```python
from build123d import *

# Parameters (mm, degrees)
SKETCH1_W                            = 26.5
SKETCH1_H                            = 6
BOSS_EXTRUDE1_DEPTH                  = 17
SKETCH2_R                            = 1.5
CUT_EXTRUDE1_DEPTH                   = 1
SKETCH3_R                            = 1.3
CUT_EXTRUDE2_DEPTH                   = 32.878676259
SKETCH4_R                            = 3
CUT_EXTRUDE3_DEPTH                   = 33.050741021
SKETCH5_R                            = 2.5
CUT_EXTRUDE4_DEPTH                   = 1.5
SKETCH6_R                            = 1.5
CUT_EXTRUDE8_DEPTH                   = 1
SKETCH7_R                            = 1.3
CUT_EXTRUDE9_DEPTH                   = 32.678068123
CUT_EXTRUDE10_START                  = -1
SKETCH8_R                            = 2.5
CUT_EXTRUDE10_DEPTH                  = 1
CUT_EXTRUDE11_START                  = -1
SKETCH9_R                            = 1.5
CUT_EXTRUDE11_DEPTH                  = 1
SKETCH10_R                           = 5.5
SKETCH10_R_2                         = 3
BOSS_EXTRUDE2_DEPTH                  = 3.5
SKETCH11_R                           = 3
SKETCH11_R_2                         = 1.3
BOSS_EXTRUDE4_DEPTH                  = 2
CUT_EXTRUDE12_START                  = -1
SKETCH12_R                           = 1.5
CUT_EXTRUDE12_DEPTH                  = 1
SKETCH17_W                           = 2
SKETCH17_H                           = 6
BOSS_EXTRUDE6_DEPTH                  = 1.5
SKETCH18_R                           = 1
CUT_EXTRUDE17_DEPTH                  = 33.050741021
CHAMFER2_SIZE                        = 5
CHAMFER2_SIZE2                       = 3.5
FILLET11_R                           = 3
BOSS_EXTRUDE7_DEPTH                  = 2
CUT_EXTRUDE19_DEPTH                  = 33.050741021
FILLET13_R                           = 5
FILLET14_R                           = 3
FILLET15_R                           = 3
SKIZZE1_R                            = 1
SCHNITT_LINEAR_AUSTRAGEN1_DEPTH      = 33.050741021
SCHNITT_LINEAR_AUSTRAGEN2_DEPTH      = 31.409702399
SCHNITT_LINEAR_AUSTRAGEN2_DEPTH_BACK = 31.409702399
SKIZZE2_W                            = 26.5
SKIZZE2_H                            = 3


with BuildPart() as part:
    # Sketch1 → Boss-Extrude1 (new body)
    with BuildSketch(Plane(origin=(0, 0, 0), x_dir=(1, 0, 0), z_dir=(0, 1, 0))):
        with Locations((13.25, 3)):
            Rectangle(SKETCH1_W, SKETCH1_H)
    extrude(amount=BOSS_EXTRUDE1_DEPTH)

    # Sketch2 → Cut-Extrude1 (cut)
    with BuildSketch(Plane.XY):
        with Locations((12.5, 5.5)):
            Circle(SKETCH2_R)
    extrude(amount=-CUT_EXTRUDE1_DEPTH, mode=Mode.SUBTRACT)

    # Sketch3 → Cut-Extrude2 (cut, through all)
    with BuildSketch(Plane.XY.offset(-1)):
        with Locations((12.5, 5.5)):
            Circle(SKETCH3_R)
    extrude(amount=-CUT_EXTRUDE2_DEPTH, mode=Mode.SUBTRACT)

    # Sketch4 → Cut-Extrude3 (cut, through all)
    with BuildSketch(Plane.XY):
        with Locations((19.208203932, 11.5)):
            Circle(SKETCH4_R)
    extrude(amount=-CUT_EXTRUDE3_DEPTH, mode=Mode.SUBTRACT)

    # Sketch5 → Cut-Extrude4 (cut)
    with BuildSketch(Plane.XY):
        with Locations((3.5, 5.5)):
            Circle(SKETCH5_R)
    extrude(amount=-CUT_EXTRUDE4_DEPTH, mode=Mode.SUBTRACT)

    # Sketch6 → Cut-Extrude8 (cut)
    with BuildSketch(Plane.XY.offset(-1.5)):
        with Locations((3.5, 5.5)):
            Circle(SKETCH6_R)
    extrude(amount=-CUT_EXTRUDE8_DEPTH, mode=Mode.SUBTRACT)

    # Sketch7 → Cut-Extrude9 (cut, through all)
    with BuildSketch(Plane.XY.offset(-2.5)):
        with Locations((3.5, 5.5)):
            Circle(SKETCH7_R)
    extrude(amount=-CUT_EXTRUDE9_DEPTH, mode=Mode.SUBTRACT)

    # Sketch8 → Cut-Extrude10 (cut)
    with BuildSketch(Plane(origin=(0, 0, -6), x_dir=(-1, 0, 0), z_dir=(0, 0, -1)).offset(CUT_EXTRUDE10_START)):
        with Locations(Location((-3.5, 5.5, 0), (0, 0, 180))):
            Circle(SKETCH8_R)
    extrude(amount=CUT_EXTRUDE10_DEPTH, mode=Mode.SUBTRACT)

    # Sketch9 → Cut-Extrude11 (cut)
    with BuildSketch(Plane(origin=(0, 0, -5), x_dir=(-1, 0, 0), z_dir=(0, 0, -1)).offset(CUT_EXTRUDE11_START)):
        with Locations(Location((-3.5, 5.5, 0), (0, 0, 180))):
            Circle(SKETCH9_R)
    extrude(amount=CUT_EXTRUDE11_DEPTH, mode=Mode.SUBTRACT)

    # Sketch10 → Boss-Extrude2 (add)
    with BuildSketch(Plane(origin=(0, 0, -6), x_dir=(-1, 0, 0), z_dir=(0, 0, -1))):
        with Locations(Location((-19.208203932, 11.5, 0), (0, 0, 90))):
            Circle(SKETCH10_R)
        with Locations(Location((-19.208203932, 11.5, 0), (0, 0, 180))):
            Circle(SKETCH10_R_2, mode=Mode.SUBTRACT)
    extrude(amount=BOSS_EXTRUDE2_DEPTH)

    # Sketch11 → Boss-Extrude4 (add)
    with BuildSketch(Plane(origin=(0, 0, -6), x_dir=(-1, 0, 0), z_dir=(0, 0, -1))):
        with Locations(Location((-12.5, 5.5, 0), (0, 0, 180))):
            Circle(SKETCH11_R)
        with Locations(Location((-12.5, 5.5, 0), (0, 0, 180))):
            Circle(SKETCH11_R_2, mode=Mode.SUBTRACT)
    extrude(amount=BOSS_EXTRUDE4_DEPTH)

    # Sketch12 → Cut-Extrude12 (cut)
    with BuildSketch(Plane(origin=(0, 0, -8), x_dir=(-1, 0, 0), z_dir=(0, 0, -1)).offset(CUT_EXTRUDE12_START)):
        with Locations(Location((-12.5, 5.5, 0), (0, 0, 180))):
            Circle(SKETCH12_R)
    extrude(amount=CUT_EXTRUDE12_DEPTH, mode=Mode.SUBTRACT)

    # Sketch17 → Boss-Extrude6 (add)
    with BuildSketch(Plane.XZ):
        with Locations((6, -3)):
            Rectangle(SKETCH17_W, SKETCH17_H)
        with Locations((20.5, -3)):
            Rectangle(SKETCH17_W, SKETCH17_H)
    extrude(amount=BOSS_EXTRUDE6_DEPTH)

    # Sketch18 → Cut-Extrude17 (cut, through all)
    with BuildSketch(Plane(origin=(0, 0, -6), x_dir=(-1, 0, 0), z_dir=(0, 0, -1))):
        with Locations((-22.5, 0)):
            Circle(SKETCH18_R)
        with Locations((-18.5, 0)):
            Circle(SKETCH18_R)
        with Locations((-8, 0)):
            Circle(SKETCH18_R)
        with Locations((-4, 0)):
            Circle(SKETCH18_R)
    extrude(amount=-CUT_EXTRUDE17_DEPTH, mode=Mode.SUBTRACT)

    # Chamfer2
    chamfer2_edges = [part.edges().sort_by_distance(p)[0] for p in [
        (26.5, 17, -3),
    ]]
    chamfer2_side = [part.faces().sort_by_distance(p)[0] for p in [
        (26.5, 8.5, -3),
    ]]
    chamfer(chamfer2_edges, length=CHAMFER2_SIZE, length2=CHAMFER2_SIZE2, reference=chamfer2_side[0])

    # Fillet11
    fillet11_edges = [part.edges().sort_by_distance(p)[0] for p in [
        (23, 17, -3),
        (26.5, 12, -3),
    ]]
    fillet(fillet11_edges, radius=FILLET11_R)

    # Sketch19 → Boss-Extrude7 (add)
    with BuildSketch(Plane(origin=(0, 0, -6), x_dir=(-1, 0, 0), z_dir=(0, 0, -1))):
        with BuildLine():
            Line((-14.547099294, 14.419606745), (-9.957579288, 7.09251277))
            ThreePointArc((-9.957579288, 7.09251277), (-14.736067977, 7.5), (-13.800160725, 2.796376119))
            Line((-13.800160725, 2.796376119), (-21.591831928, 6.543356218))
            ThreePointArc((-21.591831928, 6.543356218), (-15.108745974, 7.833333333), (-14.547099294, 14.419606745))
        make_face()
    extrude(amount=BOSS_EXTRUDE7_DEPTH)

    # Sketch20 → Cut-Extrude19 (cut, through all)
    with BuildSketch(Plane(origin=(0, 0, -6), x_dir=(-1, 0, 0), z_dir=(0, 0, -1))):
        Polygon((0, 17), (-14.011012575, 17), (-9, 9), (0, 9), align=None)
    extrude(amount=-CUT_EXTRUDE19_DEPTH, mode=Mode.SUBTRACT)

    # Fillet13
    fillet13_edges = [part.edges().sort_by_distance(p)[0] for p in [
        (14.011012575, 17, -3),
    ]]
    fillet(fillet13_edges, radius=FILLET13_R)

    # Fillet14
    fillet14_edges = [part.edges().sort_by_distance(p)[0] for p in [
        (9, 9, -3),
    ]]
    fillet(fillet14_edges, radius=FILLET14_R)

    # Fillet15
    fillet15_edges = [part.edges().sort_by_distance(p)[0] for p in [
        (0, 9, -3),
    ]]
    fillet(fillet15_edges, radius=FILLET15_R)

    # Skizze1 → Schnitt-Linear austragen1 (cut, through all)
    with BuildSketch(Plane(origin=(0, 0, -6), x_dir=(-1, 0, 0), z_dir=(0, 0, -1))):
        with Locations((-23.5, 4)):
            Circle(SKIZZE1_R)
        with Locations((-7.5, 4)):
            Circle(SKIZZE1_R)
    extrude(amount=-SCHNITT_LINEAR_AUSTRAGEN1_DEPTH, mode=Mode.SUBTRACT)

    # Skizze2 → Schnitt-Linear austragen2 (cut, two sides: drawn at the far end of the back side and taken through both)
    with BuildSketch(Plane(origin=(0, 5.5, 0), x_dir=(1, 0, 0), z_dir=(0, 1, 0)).offset(-SCHNITT_LINEAR_AUSTRAGEN2_DEPTH_BACK)):
        with Locations((13.25, 1.5)):
            Rectangle(SKIZZE2_W, SKIZZE2_H)
    extrude(amount=SCHNITT_LINEAR_AUSTRAGEN2_DEPTH + SCHNITT_LINEAR_AUSTRAGEN2_DEPTH_BACK, mode=Mode.SUBTRACT)


solid = part.part
```
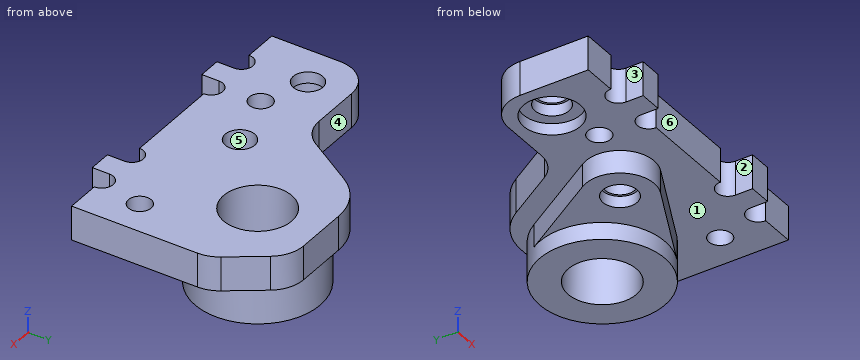
Can you work these out from the model? Positions are in its coordinate system, mm. Face numbers are marked on the shaded views. A direction names the side the tool comes from. Coordinates: 2 decimals unless noted, no trailing zeros. Order: outer loops, then holes, each group sorted by start corner. A loop starts at its lowest first (then second) coordinate and runs counter-clockwise, first axis right, second up. Notation, with made-up numbers: (14, 51.5) -> (28, 51.5) arc R28 ccw to (28, 72.5) -> close; hole circle Ø7 at (-27, -27). An arc over 180 degrees is marked (long way). Write each question's results on one line, items separated by ' | '.
Item 1: Which directions (+Z, -Z, +X, -X, +Y, -Y) give clear straight access to the entire face, cutting with the end or side of a thin tool? Please do the marked faces 1, 2 and 3.
Results are:
face 1: -Z | face 2: +Z, -Z, -Y | face 3: +Z, -Z, -X, -Y
Item 2: If I drill on line 1 along Z through (x, y) = (16.5, 2.5); line 2 along X through (y, z) = (10.25, -3.25); line 3 along Z through (x, y) = (5.25, 4), over which ranges is the centre line in solid material (lowest first)?
Results are:
line 1: -6 to -3 | line 2: 9.78 to 16.48, 21.94 to 26.5 | line 3: -5 to -3
Item 3: If we mould it in two halves opening along Y, with no side actions, what happens to the marked faces 4, 5 and 6? For each: +Y half, -Y half, draft (parallel to the pull), parting line (faces both ways), or undercut.
Results are:
face 4: +Y half | face 5: undercut | face 6: -Y half
Item 4: I'm going to push flat-ended pins straight in: pin 1 Ø1.2 at (y, z) = (-0.5, -4.5) entering from +X; pin 2 Ø2.5 at (x, y) = (2.5, 6.5) entering from -Z; pin 3 Ø0.9 at (x, y) = (12.5, 5) entering from -Z; pin 4 Ø2.5 at (x, z) = (11.5, -4) entering from -Y. Where does each tip first touch, or does it pass through?
Results are:
pin 1: x = 26.5 | pin 2: z = -6 | pin 3: through | pin 4: y = 0
Item 5: I want a section at B-B, the plane x = 4. Write out the boundary of the cut face in (y, z), then the cut area to 3 significant figures.
Results are:
outline: (1, -6) -> (3.05, -6) -> (3.05, -5) -> (4.09, -5) -> (4.09, -4) -> (4.3, -4) -> (4.3, -3) -> (1, -3) -> close; (6.7, -4) -> (6.91, -4) -> (6.91, -5) -> (7.95, -5) -> (7.95, -6) -> (9, -6) -> (9, -3) -> (6.7, -3) -> close | area: 13.9 mm²
Item 6: I want a section at D-D, the plane y = 3.5. Write out the boundary of the cut face in (x, z).
Results are:
outline: (0, -6) -> (2, -6) -> (2, -5) -> (5, -5) -> (5, -6) -> (6.63, -6) -> (6.63, -3) -> (0, -3) -> close; (8.37, -6) -> (10.26, -6) -> (10.26, -8) -> (15.26, -8) -> (15.26, -6) -> (22.63, -6) -> (22.63, -3) -> (8.37, -3) -> close; (24.37, -6) -> (26.5, -6) -> (26.5, -3) -> (24.37, -3) -> close
Item 7: I want a section at A-A, the plane z = -3.5. Count the separate pieces of the cut face and the enclosed holes in it, then the cut area to 3 significant figures.
Results are:
separate pieces: 1 | enclosed holes: 5 | area: 301 mm²
Item 8: I want a section at C-C, the plane y = 10.75. Write out the boundary of the cut face in (x, z), then the cut area to 3 significant figures.
Results are:
outline: (10.1, -6) -> (12.25, -6) -> (12.25, -8) -> (13.76, -8) -> (13.76, -9.5) -> (16.3, -9.5) -> (16.3, -3) -> (10.1, -3) -> close; (22.11, -9.5) -> (24.66, -9.5) -> (24.66, -6) -> (26.5, -6) -> (26.5, -3) -> (22.11, -3) -> close | area: 52.6 mm²
